```python
from build123d import *

# Parameters (mm, degrees)
BOSS_EXTRUDE1_DEPTH = 1.524


with BuildPart() as part:
    # Sketch1 → Boss-Extrude1 (new body)
    with BuildSketch(Plane.XY):
        with BuildLine():
            Line((-80.678958716, -0.762), (-80.678958716, -1.524))
            Line((-80.678958716, -1.524), (-78.692395213, -1.524))
            ThreePointArc((-78.692395213, -1.524), (-80.119170164, -4.335621645), (-82.784103237, -6.02056519))
            ThreePointArc((-82.784103237, -6.02056519), (-86.955126255, -5.857190971), (-90.544084344, -3.725641304))
            ThreePointArc((-90.544084344, -3.725641304), (-93.110836317, -3.021062409), (-95.425262377, -4.335626641))
            ThreePointArc((-95.425262377, -4.335626641), (-96.090143572, -4.970756046), (-96.773276943, -5.586211293))
            ThreePointArc((-96.773276943, -5.586211293), (-97.784617842, -7.488047423), (-98.148581764, -9.611092724))
            ThreePointArc((-98.148581764, -9.611092724), (-99.181314776, -8.914327019), (-99.479737369, -7.704796582))
            ThreePointArc((-99.479737369, -7.704796582), (-102.262807493, -9.439979809), (-105.21119287, -10.876421181))
            ThreePointArc((-105.21119287, -10.876421181), (-106.91403356, -12.226062588), (-108.305450104, -13.894941956))
            ThreePointArc((-108.305450104, -13.894941956), (-108.413080528, -12.98188304), (-108.807060537, -12.151196188))
            ThreePointArc((-108.807060537, -12.151196188), (-111.729155507, -12.842858899), (-114.703828793, -13.253169951))
            ThreePointArc((-114.703828793, -13.253169951), (-115.819933123, -13.705232404), (-116.747990814, -14.472538249))
            ThreePointArc((-116.747990814, -14.472538249), (-117.190021542, -13.789583851), (-117.891000612, -13.376732524))
            ThreePointArc((-117.891000612, -13.376732524), (-120.590758029, -13.228581749), (-123.267868738, -12.849481471))
            ThreePointArc((-123.267868738, -12.849481471), (-123.990419129, -13.559319569), (-124.428575307, -14.472538249))
            ThreePointArc((-124.428575307, -14.472538249), (-125.32839078, -13.121289449), (-126.552690184, -12.05515992))
            ThreePointArc((-126.552690184, -12.05515992), (-127.525021572, -11.746786856), (-128.486859712, -11.407096306))
            ThreePointArc((-128.486859712, -11.407096306), (-131.218641373, -10.554840596), (-131.89233577, -7.773634616))
            ThreePointArc((-131.89233577, -7.773634616), (-135.917529766, 7.745683618), (-146.180659468, 20.063134404))
            ThreePointArc((-146.180659468, 20.063134404), (-147.307798591, 21.249069948), (-147.538428831, 22.868852467))
            ThreePointArc((-147.538428831, 22.868852467), (-154.433810452, 31.715414423), (-159.483026723, 41.731070227))
            ThreePointArc((-159.483026723, 41.731070227), (-164.057778752, 44.14499505), (-169.123893732, 45.188962572))
            ThreePointArc((-169.123893732, 45.188962572), (-169.613633215, 45.467140142), (-169.695148012, 46.024439755))
            ThreePointArc((-169.695148012, 46.024439755), (-168.84624225, 46.858034119), (-167.67211669, 46.665811009))
            ThreePointArc((-167.67211669, 46.665811009), (-162.988364111, 45.736856959), (-158.304611532, 46.665811009))
            ThreePointArc((-158.304611532, 46.665811009), (-157.376988383, 46.865370886), (-156.791979775, 46.118327526))
            ThreePointArc((-156.791979775, 46.118327526), (-156.141187023, 44.363429515), (-156.791979775, 42.608531504))
            ThreePointArc((-156.791979775, 42.608531504), (-154.321595691, 40.375345287), (-152.040654012, 37.948985202))
            ThreePointArc((-152.040654012, 37.948985202), (-151.707852276, 38.902874077), (-151.688853759, 39.9129731))
            ThreePointArc((-151.688853759, 39.9129731), (-150.771869741, 38.327385628), (-150.840091724, 36.497005044))
            ThreePointArc((-150.840091724, 36.497005044), (-148.311639905, 32.912883943), (-146.180659468, 29.07909795))
            ThreePointArc((-146.180659468, 29.07909795), (-145.280256751, 29.950524174), (-144.888474533, 31.140740714))
            ThreePointArc((-144.888474533, 31.140740714), (-144.809080792, 29.152180218), (-145.336243225, 27.233124206))
            ThreePointArc((-145.336243225, 27.233124206), (-144.799576526, 25.915962426), (-144.308931698, 24.580974055))
            ThreePointArc((-144.308931698, 24.580974055), (-142.066206257, 22.868864738), (-141.767740402, 20.063146675))
            ThreePointArc((-141.767740402, 20.063146675), (-140.574422381, 19.11655359), (-139.418496756, 18.124645168))
            ThreePointArc((-139.418496756, 18.124645168), (-138.882087848, 18.686270696), (-138.666940721, 19.432507564))
            ThreePointArc((-138.666940721, 19.432507564), (-138.402251182, 18.434511119), (-138.666940721, 17.436514673))
            ThreePointArc((-138.666940721, 17.436514673), (-136.72060571, 15.475055994), (-134.91620317, 13.382289501))
            ThreePointArc((-134.91620317, 13.382289501), (-134.269462496, 13.942240539), (-133.926062208, 14.725754998))
            ThreePointArc((-133.926062208, 14.725754998), (-133.856105481, 13.639249521), (-134.361203786, 12.674747683))
            ThreePointArc((-134.361203786, 12.674747683), (-132.981359798, 10.757644416), (-131.718603375, 8.761472935))
            ThreePointArc((-131.718603375, 8.761472935), (-130.994013595, 9.278385285), (-130.576166715, 10.064281405))
            ThreePointArc((-130.576166715, 10.064281405), (-130.688633828, 8.984081435), (-131.3478244, 8.120977377))
            ThreePointArc((-131.3478244, 8.120977377), (-129.923570985, 5.358468693), (-128.720985312, 2.492506426))
            ThreePointArc((-128.720985312, 2.492506426), (-127.945801885, 2.902637911), (-127.329634113, 3.526700773))
            ThreePointArc((-127.329634113, 3.526700773), (-127.497659552, 2.19677598), (-128.218534166, 1.066611259))
            ThreePointArc((-128.218534166, 1.066611259), (-127.742305365, -0.477350315), (-127.329634113, -2.039500643))
            ThreePointArc((-127.329634113, -2.039500643), (-127.508941307, -4.933154821), (-124.873174428, -3.725629032))
            ThreePointArc((-124.873174428, -3.725629032), (-123.596637716, -2.585576016), (-122.254131396, -1.524))
            ThreePointArc((-122.254131396, -1.524), (-121.118350406, -0.039599921), (-120.48608758, 1.71928773))
            ThreePointArc((-120.48608758, 1.71928773), (-119.861122825, 1.004984574), (-119.026219436, 0.55360195))
            ThreePointArc((-119.026219436, 0.55360195), (-116.905277713, 1.612791346), (-114.703828793, 2.492506426))
            ThreePointArc((-114.703828793, 2.492506426), (-114.347417181, 3.526700773), (-114.703828793, 4.560895121))
            ThreePointArc((-114.703828793, 4.560895121), (-113.011657325, 3.726445198), (-111.139333293, 3.493735784))
            ThreePointArc((-111.139333293, 3.493735784), (-106.83626692, 4.069231273), (-102.495682566, 3.986148614))
            ThreePointArc((-102.495682566, 3.986148614), (-102.332792834, 5.191235076), (-102.264713723, 6.405373321))
            ThreePointArc((-102.264713723, 6.405373321), (-100.962727059, 4.560895121), (-99.006554721, 3.433660057))
            ThreePointArc((-99.006554721, 3.433660057), (-96.34050231, 2.703577616), (-93.757475163, 1.71928773))
            ThreePointArc((-93.757475163, 1.71928773), (-92.060227448, 1.486006715), (-90.544083581, 2.283739511))
            ThreePointArc((-90.544083581, 2.283739511), (-87.507868111, 4.942615236), (-83.724934757, 3.536329442))
            ThreePointArc((-83.724934757, 3.536329442), (-80.783552437, 2.373141079), (-78.692395213, 0))
            Line((-78.692395213, 0), (-80.678958716, 0))
            Line((-80.678958716, 0), (-80.678958716, -0.762))
        make_face()
    extrude(amount=BOSS_EXTRUDE1_DEPTH)


solid = part.part
```
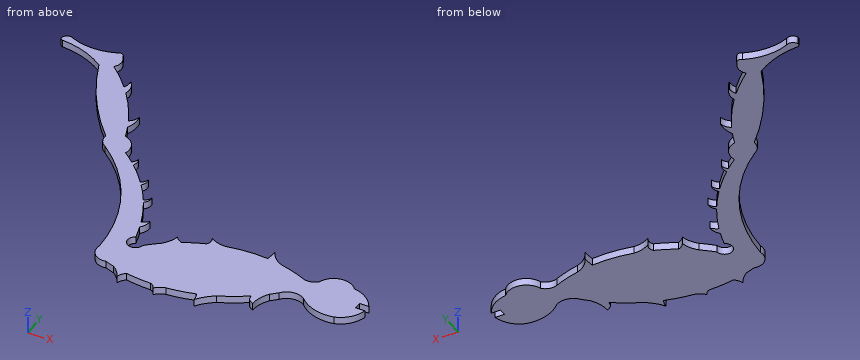
Input: part model. Units: mm. Frame: model coordinates. Coordinates: 2 decimals unless noted, no trailing zeros. Write each loop counter-clockwise with the first axis right and the second up, starting at its lowest first coordinate (ties: lowest second). Pieces come first, ordered by that corner, then holes. Notation, with made-up numbers: (82.25, -23.75) -> (129.25, -23.75) arc R28 ccw to (129.25, -2.75) -> close; hole circle Ø2 at (-25.75, -24.5). An arc over 180 degrees is marked (long way). Write each question's results on one line, items separated by ' | '.
Item 1: Section query B-B on x = -101. Return loops of the section in (y, z).
Conclusion:
outline: (-8.7, 0) -> (4.6, 0) -> (4.6, 1.52) -> (-8.7, 1.52) -> close
Item 2: Pin query (flat end, axial travel): pin 1 Ø0.5 at (x, z) = (-79.5, 0.5) entering from +Y; pin 2 Ø0.5 at (x, z) = (-80, 1) entering from -Y; pin 3 Ø2.5 at (x, y) = (-126.55, -3.54) entering from -Z. Return the tip coordinate at first contact, or that it passes through.
Conclusion:
pin 1: stops at y = 1.48 | pin 2: stops at y = -4.47 | pin 3: passes through
Item 3: Section query A-A on y = 11. Return loops of the section in (x, z).
Conclusion:
outline: (-137.8, 0) -> (-133.15, 0) -> (-133.15, 1.52) -> (-137.8, 1.52) -> close
Item 4: Material intervals for probe 1 along X at (y, z) = (-2, 0.6); probe 2 along X at (y, z) = (30, 1.25); probe 3 along Y at (x, z) = (-114, 0.9), sorted ascending.
Conclusion:
probe 1: x = -132.55 to -127.34, -122.88 to -78.81 | probe 2: x = -153.3 to -146.64, -145.25 to -144.77 | probe 3: y = -13.18 to 4.13
